Drawing for the job (mm, zero at the part's lowest x, y, z). Give positions to 0.01 mm unless a question says otherwise; leave off trailing zeros. Loops run counter-clockwise (first coordinate to the right, second up) from the corner with the lowest first, then second, coordinate; pieces in that order, holes last. Notation, with made-up numbers: (4, -3) - (29, -3) arc R33 ccw to (29, 32) - close; hole circle Ø8 at (-39, 44.25). An arc over 180 degrees is marked (long way). Return JSON: item names as keys, results as strings. Group by question number.
1) Drop a flat-ended pin along its axis: pin 1 (2 mm diameter, centred on x = 31.5, z = 25.5, fed in from -Y). Give the stop position or say it passes through.
2) Slice it at D-D (x = 29). List the corners of the cut face in (y, z).
3) Slice it at B-B (z = 33). List the corners of the cut face in (x, y), and give its area (3 significant figures).
4) Drill centre lines: probe 1 along X at (y, z) = (2.25, 4); probe 2 along X at (y, z) = (1.1, 26) (1 decimal); probe 3 along Z at (x, y) = (46, 0.85) (1 decimal). Where is each one in solid material? Low to high. Write a range as from..to.
5) Slice it at C-C (y = 0.95). List the corners of the cut face in (x, z), and give its area (3 significant figures).
6) Slice it at A-A (x = 56). List the corners of the cut face in (y, z).
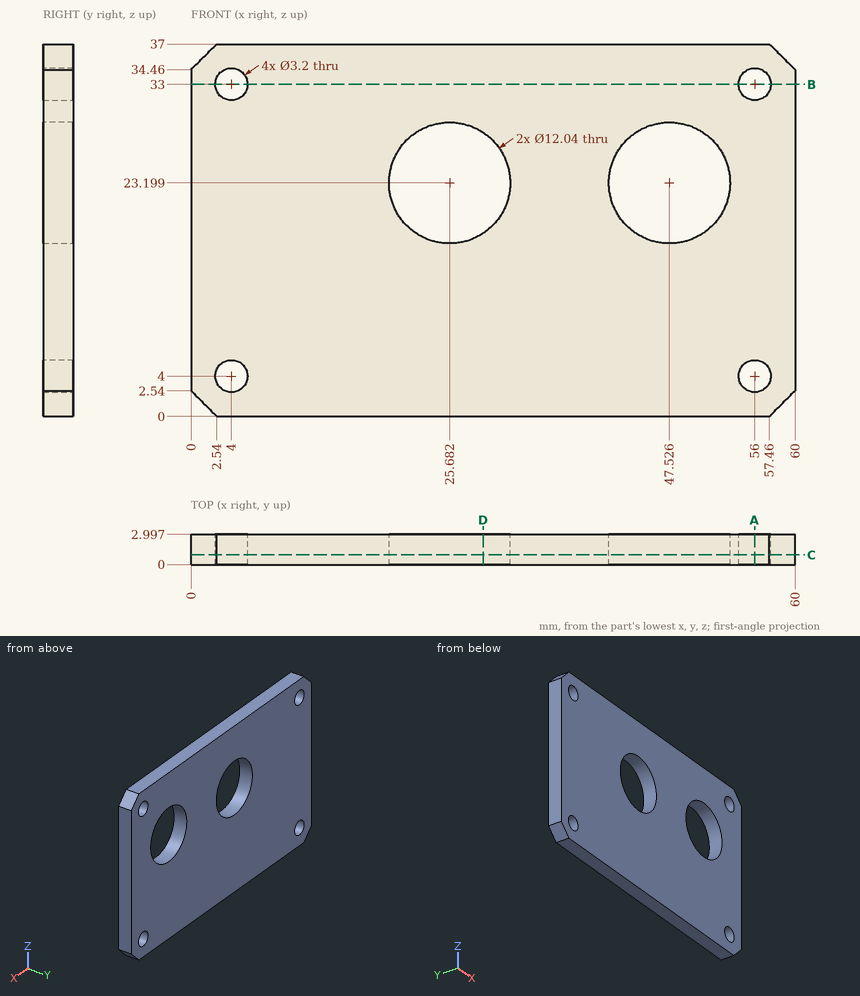
Results:
{
 "1": {"pin 1": "y = 0"},
 "2": {"outline": "(0, 0) - (3, 0) - (3, 18.18) - (0, 18.18) - close; (0, 28.22) - (3, 28.22) - (3, 37) - (0, 37) - close"},
 "3": {"outline": "(0, 0) - (2.4, 0) - (2.4, 3) - (0, 3) - close; (5.6, 0) - (54.4, 0) - (54.4, 3) - (5.6, 3) - close; (57.6, 0) - (60, 0) - (60, 3) - (57.6, 3) - close", "area": "161 mm2"},
 "4": {"probe 1": "0..2.4, 5.6..54.4, 57.6..60", "probe 2": "0..20.4, 31..42.2, 52.9..60", "probe 3": "0..17.4, 29..37"},
 "5": {"outline": "(0, 2.54) - (2.54, 0) - (57.46, 0) - (60, 2.54) - (60, 34.46) - (57.46, 37) - (2.54, 37) - (0, 34.46) - close; hole circle Ø3.2 at (4, 4); hole circle Ø3.2 at (4, 33); hole circle Ø12.04 at (25.68, 23.2); hole circle Ø12.04 at (47.53, 23.2); hole circle Ø3.2 at (56, 4); hole circle Ø3.2 at (56, 33)", "area": "1,950 mm2"},
 "6": {"outline": "(0, 0) - (3, 0) - (3, 2.4) - (0, 2.4) - close; (0, 5.6) - (3, 5.6) - (3, 31.4) - (0, 31.4) - close; (0, 34.6) - (3, 34.6) - (3, 37) - (0, 37) - close"}
}
